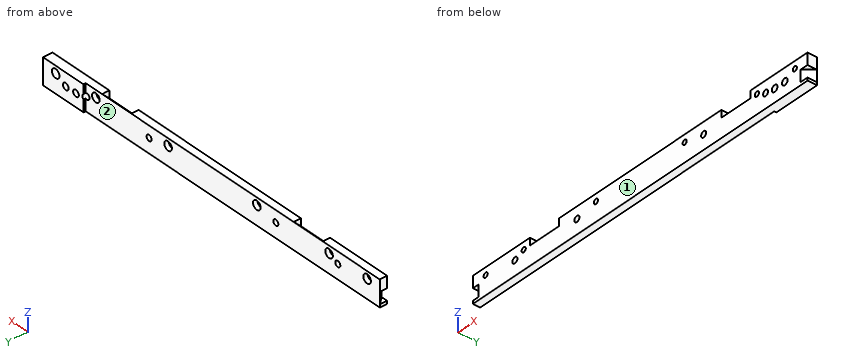
from build123d import *

# Parameters (mm, degrees)
SKIZZE1_W                       = 264
SKIZZE1_H                       = 18
SKIZZE1_R                       = 1.65
SKIZZE1_R_2                     = 2.25
SKIZZE1_R_3                     = 2
AUFSATZ_LINEAR_AUSTRAGEN1_DEPTH = 5
SCHNITT_LINEAR_START            = -2
SCHNITT_LINEAR_AUSTRAGEN1_DEPTH = 8
SCHNITT_LINEAR_START_2          = -44.9
SCHNITT_LINEAR_AUSTRAGEN2_DEPTH = 23.1
SCHNITT_LINEAR_AUSTRAGEN3_DEPTH = 23.1
SKIZZE5_R                       = 3
SCHNITT_LINEAR_AUSTRAGEN4_DEPTH = 3
SKIZZE7_W                       = 32
SKIZZE7_H                       = 18
SKIZZE7_R                       = 2.25
SKIZZE7_R_2                     = 3
AUFSATZ_LINEAR_AUSTRAGEN3_DEPTH = 1.5
AUFSATZ_LINEAR_START            = -5
SKIZZE8_R                       = 2.25
AUFSATZ_LINEAR_AUSTRAGEN4_DEPTH = 5
SCHNITT_LINEAR_AUSTRAGEN6_DEPTH = 8
SKIZZE10_R                      = 2
SCHNITT_LINEAR_AUSTRAGEN7_DEPTH = 1.5


with BuildPart() as part:
    # Skizze1 → Aufsatz-Linear austragen1 (new body)
    with BuildSketch(Plane(origin=(0, 0, 0), x_dir=(1, 0, 0), z_dir=(0, 1, 0))):
        with Locations((132, 9)):
            Rectangle(SKIZZE1_W, SKIZZE1_H)
        with Locations(Location((10, 5, 0), (0, 0, 270))):
            Circle(SKIZZE1_R, mode=Mode.SUBTRACT)
        with Locations(Location((40, 5, 0), (0, 0, 270))):
            Circle(SKIZZE1_R, mode=Mode.SUBTRACT)
        with Locations(Location((26, 9, 0), (0, 0, 270))):
            Circle(SKIZZE1_R_2, mode=Mode.SUBTRACT)
        with Locations(Location((18, 9, 0), (0, 0, 270))):
            Circle(SKIZZE1_R_2, mode=Mode.SUBTRACT)
        with Locations(Location((224, 5, 0), (0, 0, 90))):
            Circle(SKIZZE1_R, mode=Mode.SUBTRACT)
        with Locations(Location((254, 5, 0), (0, 0, 90))):
            Circle(SKIZZE1_R, mode=Mode.SUBTRACT)
        with Locations(Location((246, 9, 0), (0, 0, 90))):
            Circle(SKIZZE1_R_2, mode=Mode.SUBTRACT)
        with Locations(Location((238, 9, 0), (0, 0, 90))):
            Circle(SKIZZE1_R_2, mode=Mode.SUBTRACT)
        with Locations(Location((230.9, 8, 0), (0, 0, 90))):
            Circle(SKIZZE1_R_3, mode=Mode.SUBTRACT)
        with Locations(Location((33.1, 8, 0), (0, 0, 270))):
            Circle(SKIZZE1_R_3, mode=Mode.SUBTRACT)
        with Locations(Location((97, 5, 0), (0, 0, 270))):
            Circle(SKIZZE1_R, mode=Mode.SUBTRACT)
        with Locations(Location((167, 5, 0), (0, 0, 270))):
            Circle(SKIZZE1_R, mode=Mode.SUBTRACT)
        with Locations(Location((82, 8, 0), (0, 0, 270))):
            Circle(SKIZZE1_R_3, mode=Mode.SUBTRACT)
        with Locations(Location((182, 8, 0), (0, 0, 270))):
            Circle(SKIZZE1_R_3, mode=Mode.SUBTRACT)
    extrude(amount=AUFSATZ_LINEAR_AUSTRAGEN1_DEPTH)

    # Skizze2 → Schnitt-Linear austragen1 (cut)
    with BuildSketch(Plane(origin=(0, 0, -18), x_dir=(-1, 0, 0), z_dir=(0, 0, -1)).offset(SCHNITT_LINEAR_START)):
        Polygon((-4.195498156, 0), (0, 0), (0, 5), align=None)
        Polygon((-264, 0), (-259.804501844, 0), (-264, 5), align=None)
    extrude(amount=-SCHNITT_LINEAR_AUSTRAGEN1_DEPTH, mode=Mode.SUBTRACT)

    # Skizze3 → Schnitt-Linear austragen2 (cut)
    with BuildSketch(Plane.ZY.offset(SCHNITT_LINEAR_START_2)):
        Polygon((0, 5), (-5, 0), (0, 0), align=None)
    extrude(amount=-SCHNITT_LINEAR_AUSTRAGEN2_DEPTH, mode=Mode.SUBTRACT)

    # Skizze4 → Schnitt-Linear austragen3 (cut)
    with BuildSketch(Plane(origin=(264, 0, 0), x_dir=(0, 0, -1), z_dir=(1, 0, 0)).offset(SCHNITT_LINEAR_START_2)):
        Polygon((0, 5), (5, 0), (0, 0), align=None)
    extrude(amount=-SCHNITT_LINEAR_AUSTRAGEN3_DEPTH, mode=Mode.SUBTRACT)

    # Skizze5 → Schnitt-Linear austragen4 (cut)
    with BuildSketch(Plane(origin=(0, 5, 0), x_dir=(1, 0, 0), z_dir=(0, 1, 0))):
        with Locations(Location((254, 5, 0), (0, 0, 270))):
            Circle(SKIZZE5_R)
        with Locations(Location((224, 5, 0), (0, 0, 270))):
            Circle(SKIZZE5_R)
        with Locations(Location((40, 5, 0), (0, 0, 270))):
            Circle(SKIZZE5_R)
        with Locations(Location((10, 5, 0), (0, 0, 270))):
            Circle(SKIZZE5_R)
        with Locations(Location((97, 5, 0), (0, 0, 270))):
            Circle(SKIZZE5_R)
        with Locations(Location((167, 5, 0), (0, 0, 270))):
            Circle(SKIZZE5_R)
    extrude(amount=-SCHNITT_LINEAR_AUSTRAGEN4_DEPTH, mode=Mode.SUBTRACT)

    # Skizze7 → Aufsatz-Linear austragen3 (add)
    with BuildSketch(Plane(origin=(0, 5, 0), x_dir=(1, 0, 0), z_dir=(0, 1, 0))):
        with Locations((248, 9)):
            Rectangle(SKIZZE7_W, SKIZZE7_H)
        with Locations(Location((238, 9, 0), (0, 0, 90))):
            Circle(SKIZZE7_R, mode=Mode.SUBTRACT)
        with Locations(Location((246, 9, 0), (0, 0, 90))):
            Circle(SKIZZE7_R, mode=Mode.SUBTRACT)
        with Locations(Location((254, 5, 0), (0, 0, 270))):
            Circle(SKIZZE7_R_2, mode=Mode.SUBTRACT)
    extrude(amount=AUFSATZ_LINEAR_AUSTRAGEN3_DEPTH)

    # Skizze8 → Aufsatz-Linear austragen4 (add)
    with BuildSketch(Plane(origin=(0, 5, 0), x_dir=(1, 0, 0), z_dir=(0, 1, 0)).offset(AUFSATZ_LINEAR_START)):
        with Locations((18, 9)):
            Circle(SKIZZE8_R)
        with Locations((26, 9)):
            Circle(SKIZZE8_R)
    extrude(amount=AUFSATZ_LINEAR_AUSTRAGEN4_DEPTH)

    # Skizze9 → Schnitt-Linear austragen6 (cut)
    with BuildSketch(Plane(origin=(0, 0, -18), x_dir=(-1, 0, 0), z_dir=(0, 0, -1)).offset(SCHNITT_LINEAR_START)):
        Polygon((-264, 6.5), (-264, 0), (-258.545852397, 0), align=None)
    extrude(amount=-SCHNITT_LINEAR_AUSTRAGEN6_DEPTH, mode=Mode.SUBTRACT)

    # Skizze10 → Schnitt-Linear austragen7 (cut)
    with BuildSketch(Plane(origin=(0, 5, 0), x_dir=(1, 0, 0), z_dir=(0, 1, 0))):
        with Locations(Location((230.9, 8, 0), (0, 0, 90))):
            Circle(SKIZZE10_R)
    extrude(amount=SCHNITT_LINEAR_AUSTRAGEN7_DEPTH, mode=Mode.SUBTRACT)


solid = part.part
Can you work these out from the model? Positions are in its coordinate system, mm. Face numbers are marked on the shaded views. A direction names the side the tool comes from. Coordinates: 2 decimals unless noted, no trailing zeros. Write each loop counter-clockwise with the first axis right and the second up, starting at its lowest first coordinate (ties: lowest second). Pieces come first, ordered by that corner, then holes.
Q1. For P1, Ø0.8, axis at y = 6, z = -2.5, coming from the -X side; P2, Ø3, axis at x = 10.5, z = -6, coming from the +Y side; P3, Ø6.5, axis at x = 96.5, z = -4.5, coming from the +Y side, each with a flat end and sliding along its axis, tell me the tip position at first contact or that it passes through.
Results found:
P1: stops at x = 232
P2: stops at y = 2
P3: stops at y = 5
Q2. Imagine slicing it at B-B, the plane y = 4. Count the separate pieces of the cut face and the enclosed holes in it, plus the area to 3 significant figures.
Results found:
separate pieces: 1
enclosed holes: 12
area: 4,430 mm2
Q3. Please list where these lines run through material, in increasing order: L1, parallel to Z at x = 254, y = 5.15; L2, parallel to Z at x = 238, y = 3; L3, parallel to Y at x = 28, z = -7.5.
Results found:
L1: z = -18 to -8, -2 to 0
L2: z = -18 to -11.25, -6.75 to 0
L3: y = 0 to 5
Q4. Imagine slicing it at C-C, the plane x = 21. List the corners of the cut face in (y, z) for me, plus the area to 3 significant figures.
Results found:
outline: (0, -18) - (5, -18) - (5, 0) - (0, 0) - close
area: 90.0 mm2
Q5. Which directions (+Z, -Z, +X, -X, +Y, -Y) give clear straight access to the entire face, cutting with the end or side of a thin tool? Please do the marked faces 1 and 2.
Results found:
face 1: +Z, -Z, +X, -X, -Y
face 2: +Z, -Z, -X, +Y
Q6. Imagine slicing it at A-A, the plane x = 238. List the corners of the cut face in (y, z) for me, plus the area to 4 significant figures.
Results found:
outline: (0, -18) - (6.5, -18) - (6.5, -11.25) - (0, -11.25) - close; (0, -6.75) - (6.5, -6.75) - (6.5, 0) - (0, 0) - close
area: 87.75 mm2
